Could you check a few things on this model? Use its own coordinates, in mm. Give positions to 0.01 mm unless a question says otherwise; leave off trailing zeros. Write each loop counter-clockwise with the first axis right and the second up, starting at its lowest first coordinate (ties: lowest second). Pieces come first, ordered by that corner, then holes. Notation, with made-up numbers: (-6.5, 38.5) - (5.5, 38.5) arc R30 cw to (5.5, 77.5) - close; hole circle Ø9 at (56, 3.5). An arc over 180 degrees is marked (long way). Use one line per item in the form item = value.
```python
from build123d import *

# Parameters (mm, degrees)
F0_W     = 75
F0_H     = 32
F1_DEPTH = 1
F2_R     = 2
F3_DEPTH = 25.4
F4_R     = 0.5


with BuildPart() as f1:
    # F0 (on Front) → F1 (new body, symmetric)
    with BuildSketch(Plane.XZ):
        Rectangle(F0_W, F0_H)
    extrude(amount=F1_DEPTH, both=True)

    # F2 (on face) → F3 (cut)
    with BuildSketch(Plane.XZ.offset(1)):
        with Locations((-32.5, 11)):
            Circle(F2_R)
        with Locations((-32.5, -11)):
            Circle(F2_R)
        with Locations((32.5, -11)):
            Circle(F2_R)
        with Locations((32.5, 11)):
            Circle(F2_R)
    extrude(amount=-F3_DEPTH, mode=Mode.SUBTRACT)

    # F4
    f4_edges = [f1.edges().sort_by_distance(p)[0] for p in [
        (37.5, 0, 16),
        (37.5, 0, -16),
        (-37.5, 0, 16),
        (-37.5, 0, -16),
    ]]
    fillet(f4_edges, radius=F4_R)


solid = f1.part
```
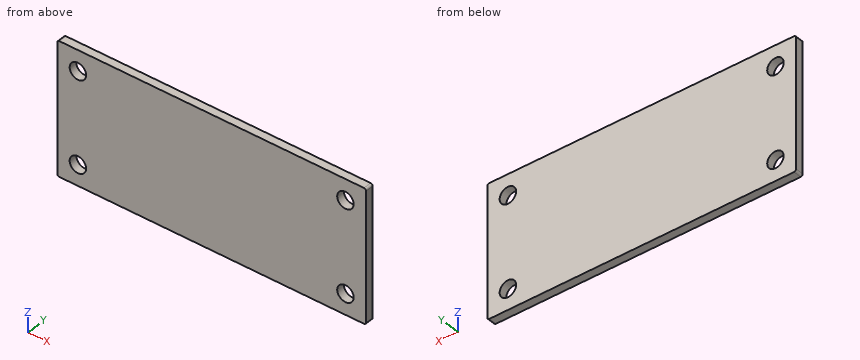
1. Imagine slicing it at A-A, the plane x = -32.5. List the corners of the cut face in (y, z) for me, and give its area (3 significant figures).
Response values:
outline = (-1, -16) - (1, -16) - (1, -13) - (-1, -13) - close; (-1, -9) - (1, -9) - (1, 9) - (-1, 9) - close; (-1, 13) - (1, 13) - (1, 16) - (-1, 16) - close
area = 48.0 mm²
2. Imagine slicing it at C-C, the plane y = 0.6. List the corners of the cut face in (x, z) for me, and give its area (3 significant figures).
Response values:
outline = (-37.5, -15.5) arc R0.5 ccw to (-37, -16) - (37, -16) arc R0.5 ccw to (37.5, -15.5) - (37.5, 15.5) arc R0.5 ccw to (37, 16) - (-37, 16) arc R0.5 ccw to (-37.5, 15.5) - close; hole circle Ø4 at (-32.5, -11); hole circle Ø4 at (-32.5, 11); hole circle Ø4 at (32.5, -11); hole circle Ø4 at (32.5, 11)
area = 2,350 mm²
3. If I drill on line 1 (Z direction, x = 32.5, y = -0.55); line 2 (Z direction, x = 33, y = 0.5); line 3 (X direction, y = 0.7, z = -10), over which ranges is the centre line in solid material (lowest first)? Write a range as from..to.
Response values:
line_1 = -16..-13, -9..9, 13..16
line_2 = -16..-12.94, -9.06..9.06, 12.94..16
line_3 = -37.5..-34.23, -30.77..30.77, 34.23..37.5
4. For pin 1 (3 mm diameter, centred on x = 32.5, z = -11, fed in from -Y), with a flat end and sliding along its axis, tell me the tip position at first contact or that it passes through.
Response values:
pin_1 = through
5. Imagine slicing it at B-B, the plane z = 11. List the corners of the cut face in (x, y) for me, and give its area (3 significant figures).
Response values:
outline = (-37.5, -1) - (-34.5, -1) - (-34.5, 1) - (-37.5, 1) - close; (-30.5, -1) - (30.5, -1) - (30.5, 1) - (-30.5, 1) - close; (34.5, -1) - (37.5, -1) - (37.5, 1) - (34.5, 1) - close
area = 134 mm²
